```python
from build123d import *

# Parameters (mm, degrees)
SKETCH1_W           = 139
SKETCH1_H           = 8.9
BOSS_EXTRUDE1_DEPTH = 4.5
SKETCH1_3_R         = 2.125
BOSS_EXTRUDE2_DEPTH = 3
CUT_EXTRUDE1_DEPTH  = 200
CUT_EXTRUDE4_DEPTH  = 200
CUT_EXTRUDE5_DEPTH  = 200
CUT_EXTRUDE6_DEPTH  = 200
CUT_EXTRUDE8_DEPTH  = 361


with BuildPart() as part:
    # Sketch1 → Boss-Extrude1 (new body, symmetric)
    with BuildSketch(Plane.XY):
        with Locations((69.5, 4.45)):
            Rectangle(SKETCH1_W, SKETCH1_H)
    extrude(amount=BOSS_EXTRUDE1_DEPTH, both=True)

    # Sketch1_3 → Boss-Extrude2 (add, symmetric)
    with BuildSketch(Plane.XY):
        with BuildLine():
            Line((0, 4.45), (0, 8.9))
            Line((0, 8.9), (0, 9.4))
            Line((0, 9.4), (-7.008929738, 9.4))
            ThreePointArc((-7.008929738, 9.4), (-8.32, 4.45), (-7.008929738, -0.5))
            Line((-7.008929738, -0.5), (0, -0.5))
            Line((0, -0.5), (0, 0))
            Line((0, 0), (0, 4.45))
        make_face()
        with Locations((-4.125, 4.45)):
            Circle(SKETCH1_3_R, mode=Mode.SUBTRACT)
    extrude(amount=BOSS_EXTRUDE2_DEPTH, both=True)

    # Sketch2 → Cut-Extrude1 (cut, symmetric)
    with BuildSketch(Plane(origin=(139, 0, 0), x_dir=(0, 0, -1), z_dir=(1, 0, 0))):
        with BuildLine():
            ThreePointArc((0.05, 8.9), (3.196625176, 7.596625176), (4.5, 4.45))
            Line((4.5, 4.45), (4.5, 8.9))
            Line((4.5, 8.9), (0.05, 8.9))
        make_face()
        with BuildLine():
            Line((4.5, 0), (4.5, 4.45))
            ThreePointArc((4.5, 4.45), (3.196625176, 1.303374824), (0.05, 0))
            Line((0.05, 0), (4.5, 0))
        make_face()
        with BuildLine():
            Line((-4.5, 0), (0.05, 0))
            ThreePointArc((0.05, 0), (-3.096625176, 1.303374824), (-4.4, 4.45))
            Line((-4.4, 4.45), (-4.5, 0))
        make_face()
        with BuildLine():
            ThreePointArc((-4.4, 4.45), (-3.096625176, 7.596625176), (0.05, 8.9))
            Line((0.05, 8.9), (-4.4, 8.9))
            Line((-4.4, 8.9), (-4.4, 4.45))
        make_face()
    extrude(amount=CUT_EXTRUDE1_DEPTH, both=True, mode=Mode.SUBTRACT)

    # Sketch5 → Cut-Extrude4 (cut, symmetric)
    with BuildSketch(Plane(origin=(0, 0, -3), x_dir=(-1, 0, 0), z_dir=(0, 0, -1))):
        Polygon((7.27530569, 8.9), (0, 8.9), (-1.536483872, 9.442626596), (6.771268728, 9.782768914), align=None)
    extrude(amount=CUT_EXTRUDE4_DEPTH, both=True, mode=Mode.SUBTRACT)

    # Sketch6 → Cut-Extrude5 (cut, symmetric)
    with BuildSketch(Plane.XY.offset(3)):
        Polygon((0, 0), (0.715891122, -1.192951857), (-7.933711104, -1.400818057), (-7.27530569, 0), align=None)
    extrude(amount=CUT_EXTRUDE5_DEPTH, both=True, mode=Mode.SUBTRACT)

    # Sketch7 → Cut-Extrude6 (cut, symmetric)
    with BuildSketch(Plane.XY.offset(3)):
        Polygon((-7.27530569, 8.9), (-6.80653665, 9.625984501), (-7.207484275, 9.625984501), align=None)
    extrude(amount=CUT_EXTRUDE6_DEPTH, both=True, mode=Mode.SUBTRACT)

    # Sketch8 → Cut-Extrude8 (cut, symmetric)
    with BuildSketch(Plane(origin=(139, 0, 0), x_dir=(0, 0, -1), z_dir=(1, 0, 0))):
        Polygon((-4.4, 4.45), (-4.497226285, 0.123430317), (-4.497226285, -0.993132251), (-5.525689044, -1.409682141), (-10.667797883, 2.280439271), (-5.525689044, 10.659843857), (-2.697341369, 11.337001628), (-4.4, 7.708140942), align=None)
    extrude(amount=CUT_EXTRUDE8_DEPTH, both=True, mode=Mode.SUBTRACT)


solid = part.part
```
The listing builds one solid part. Answer for the finished solid, in the listing's coordinates (mm). A direction names the side the tool comes from. Give positions to 0.01 mm unless a question says otherwise; leave off trailing zeros. Order: outer loops, then holes, each group sorted by start corner. A loop starts at its lowest first (then second) coordinate and runs counter-clockwise, first axis right, second up. Notation, with made-up numbers: (89.5, 53) - (129.5, 53) arc R21 ccw to (129.5, 65) - close; hole circle Ø10 at (22, 47). An arc over 180 degrees is marked (long way). Answer in a Markdown table with one row per item. Add a question column.
Q1. For a pull along X with two mould halves and no side action, classify faces 3 (the flat face through (-4, 7, 3)), 4 (the cylindrical face through (-5.811, 3.157, -0.042)), 5 (the flat face through (139, 4, 0)) as released by +X, released by -X, zero draft, split by the parting line, or undercut.
Q2. Find the intervals of material crossed by line 1 along Z through (x, y) = (133, 4); line 2 along Y through (x, z) = (71, 0.25); line 3 along Z through (x, y) = (54, 5.5), in increasing order. Write a range as [from, to].
Q3. The part is cut by section A-A (z = -1.25). Determine the outline of the cut face in (x, y) (3 decimals), then the cut area to 3 significant figures.
Q4. The part is cut by section B-B (x = 72.5). Determine the outline of the cut face in (y, z).
Q5. Which of the six approach directions +Z, -Z, +X, -X, +Y, -Y give full straight-line access (tool end or side, diameter ignored) to faces 1 (the flat face through (-4, 7, -3)), 2 (the cylindrical face through (-8.32, 4.51, 0.04))?
Q6. Given P1, Ø2, axis at x = -5.5, y = 4.5, coming from the -Z side; P2, Ø0.5, axis at y = 4.5, z = -4, coming from the -X side; P3, Ø1, axis at x = 31, y = 2, coming from the -Z side, each flat-ended and moving along its own axis, determine where each tip first touches the part or whether it passes through.
Determined:
| question | item | result |
|---|---|---|
| 1 | face 3 | zero draft |
| 1 | face 4 | undercut |
| 1 | face 5 | released by +X |
| 2 | line 1 | z = [-4.48, 4.38] |
| 2 | line 2 | y = [0.01, 8.89] |
| 2 | line 3 | z = [-4.37, 4.27] |
| 3 | outline | (-7.355, 0.165) - (139, 0.165) - (139, 8.735) - (-7.355, 8.735) arc R10 ccw to start; hole circle Ø4.25 at (-4.125, 4.45) |
| 3 | area | 1,250 mm² |
| 4 | outline | circle Ø8.9 at (4.45, -0.05) |
| 5 | face 1 | -Z, -X, +Y, -Y |
| 5 | face 2 | +Z, -Z, -X |
| 6 | P1 | stops at z = -3 |
| 6 | P2 | stops at x = 0 |
| 6 | P3 | stops at z = -4.05 |
